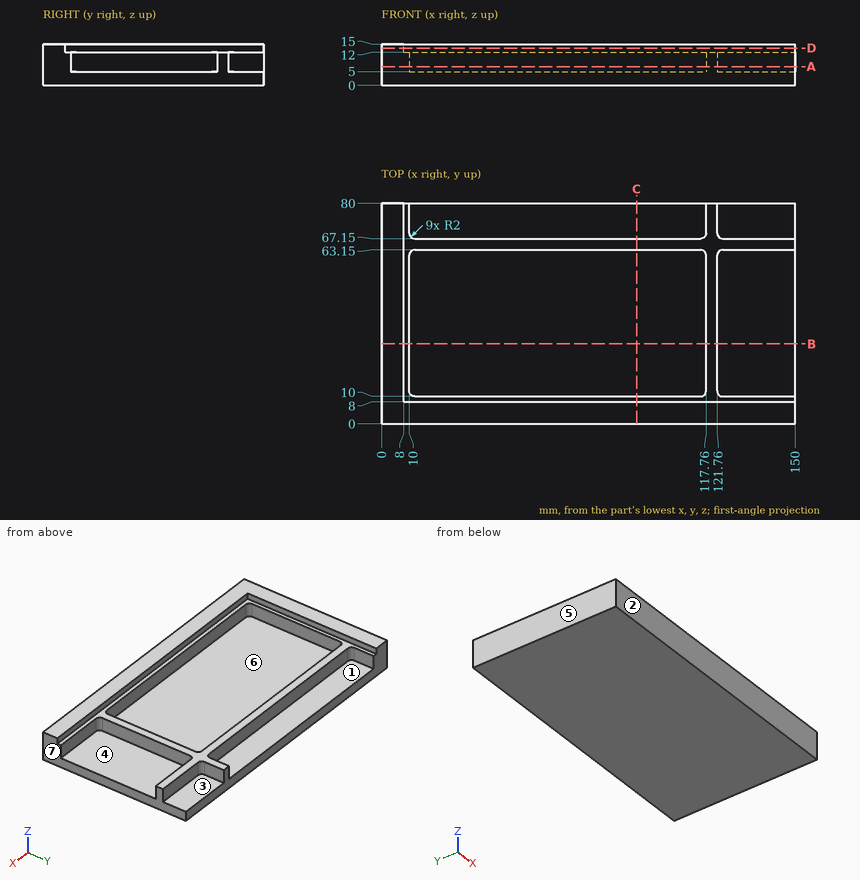
Part print with two shaded views. Sizes in mm from the minimum x, y, z corner. A direction names the side the tool comes from. Round coordinates to 2 decimals unless told otherwise and drop trailing zeros. Loops run counter-clockwise (first coordinate to the right, second up) from the corner with the lowest first, then second, coordinate; pieces in that order, holes last.
Item 1: Which spindle directions (+Z, -Z, +X, -X, +Y, -Y) get a long thin tool onto all of the face, cutting with end or side? Do the marked faces 1, 2 and 3. Say none if no direction does.
Item 2: Saw through at D-D (z = 13.5). List the corners of the cut face in (x, y).
Item 3: Saw through at A-A (z = 6.75). List the corners of the cut face in (x, y), then the cut area to 3 significant figures.
Item 4: Two-plate mould, pull along X, no slides. Class the marked faces 4, 5, 6 and 7: released by +X, released by -X, zero draft, split by the parting line, or undercut.
Item 5: Pin check, flat tips, straight feed: P1, Ø14, axis at x = 51.5, y = 75, coming from the +Z side; P2, Ø1.5, axis at y = 34, z = 13.5, coming from the +X side; P3, Ø2, axis at y = 76.5, z = 8.5, coming from the +X side. Stop position of each tip, or through.
Item 6: Saw through at C-C (x = 92.5). List the corners of the cut face in (y, z), then the cut area to 3 significant figures.
Item 7: Drill centre lines: line 1 along Y through (x, z) = (21, 10.5); line 2 along X through (y, z) = (12.5, 10.75); line 3 along Z through (x, y) = (24.5, 33.5). Where is each one in solid material? Low to high.
Item 8: Saw through at B-B (y = 29). List the corners of the cut face in (x, z), then the cut area to 3 significant figures.
Worked answers:
1. face 1: +Z, +Y
1. face 2: +Z, -Z, +X, -X, -Y
1. face 3: +Z, +X, +Y
2. outline: (0, 0) - (150, 0) - (150, 8) - (8, 8) - (8, 80) - (0, 80) - close
3. outline: (0, 0) - (150, 0) - (150, 10) - (123.76, 10) arc R2 cw to (121.76, 12) - (121.76, 61.15) arc R2 cw to (123.76, 63.15) - (150, 63.15) - (150, 67.15) - (123.76, 67.15) arc R2 cw to (121.76, 69.15) - (121.76, 80) - (117.76, 80) - (117.76, 69.15) arc R2 cw to (115.76, 67.15) - (12, 67.15) arc R2 cw to (10, 69.15) - (10, 80) - (0, 80) - close; hole (10, 12) arc R2 ccw to (12, 10) - (115.76, 10) arc R2 ccw to (117.76, 12) - (117.76, 61.15) arc R2 ccw to (115.76, 63.15) - (12, 63.15) arc R2 ccw to (10, 61.15) - close
3. area: 3,030 mm2
4. face 4: zero draft
4. face 5: released by -X
4. face 6: undercut
4. face 7: released by +X
5. P1: stops at z = 5
5. P2: stops at x = 8
5. P3: stops at x = 121.76
6. outline: (0, 0) - (80, 0) - (80, 5) - (67.15, 5) - (67.15, 12) - (63.15, 12) - (63.15, 5) - (10, 5) - (10, 12) - (8, 12) - (8, 15) - (0, 15) - close
6. area: 522 mm2
7. line 1: y = 0 to 10, 63.15 to 67.15
7. line 2: x = 0 to 10, 117.76 to 121.76
7. line 3: z = 0 to 5
8. outline: (0, 0) - (150, 0) - (150, 5) - (121.76, 5) - (121.76, 12) - (117.76, 12) - (117.76, 5) - (10, 5) - (10, 12) - (8, 12) - (8, 15) - (0, 15) - close
8. area: 872 mm2
